For this review, take the finished solid that the model builds, in its own axes (mm). Face numbers are marked on the shaded views. Round coordinates to 2 decimals unless told otherwise and drop trailing zeros. Order: outer loops, then holes, each group sorted by start corner. A loop starts at its lowest first (then second) coordinate and runs counter-clockwise, first axis right, second up. Notation, with made-up numbers: (82.25, -9) -> (135.25, -9) arc R15 ccw to (135.25, -3) -> close; hole circle Ø9 at (83.5, 88.25). An arc over 180 degrees is marked (long way). Use a Markdown table: item, result. Add a question column.
1) Wall thickness on line 1 along X through (y, z) = (8, 0); line 2 along X through (y, z) = (8.75, 43); line 3 along X through (y, z) = (9, 0): over which ranges is each line inside the solid? List them lowest first. Write a range as [from, to].
2) Draft analysis for pull direction Z (two halves, no side actions). For the marked faces 1 and 2, state which applies: pulls with the +Z half, pulls with the -Z half, needs draft (parallel to the pull), parting line crosses it, or undercut.
3) Consider section A-A (x = 0). State the section outline as (y, z) points, plus the area to 3 significant figures.
4) Clearance check with flat-ended pins moving along their axes: P1, Ø5.5, axis at x = 72.5, y = 12.5, coming from the -Z side; P2, Ø5, axis at x = 16.5, y = 13.5, coming from the +Z side; P3, Ø5, axis at x = -97, z = 46.5, coming from the +Y side. State where each tip first meets the part, or that it passes through.
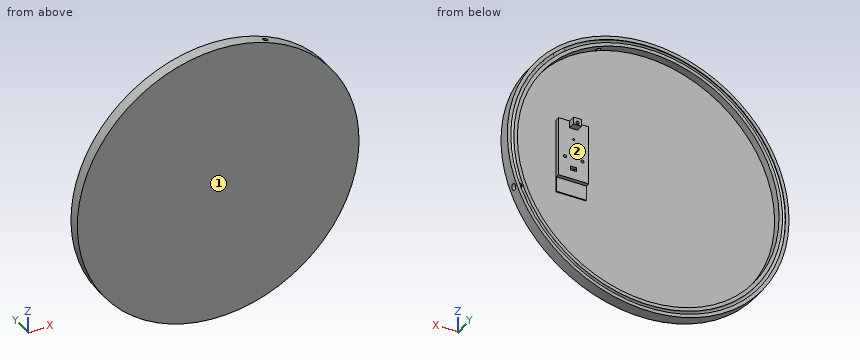
```python
from build123d import *

# Parameters (mm, degrees)
SKETCH1_R                 = 141
BOSS_EXTRUDE1_DEPTH       = 3.5
SKETCH2_R                 = 141
SKETCH2_R_2               = 131
BOSS_EXTRUDE2_DEPTH       = 8
SKETCH5_R                 = 2
CUT_EXTRUDE3_DEPTH        = 5
CUT_EXTRUDE3_DEPTH_BACK   = 15
SKETCH7_W                 = 30
SKETCH7_H                 = 75
SKETCH7_R                 = 1
BOSS_EXTRUDE3_DEPTH       = 5
SKETCH8_W                 = 8
SKETCH8_H                 = 7
BOSS_EXTRUDE4_DEPTH       = 7
SKETCH9_W                 = 6
SKETCH9_H                 = 4
CUT_EXTRUDE6_DEPTH        = 3.5
F_3_0MM_DOWEL_HOLE2_D     = 3
F_3_0MM_DOWEL_HOLE2_DEPTH = 10
F_3_0MM_DOWEL_HOLE2_TIP   = 0.901290929
F_3_0MM_DOWEL_HOLE3_D     = 3
F_3_0MM_DOWEL_HOLE3_DEPTH = 5
F_3_0MM_DOWEL_HOLE3_TIP   = 0.901290929
SKETCH10_W                = 30
SKETCH10_H                = 15
CUT_EXTRUDE7_DEPTH        = 4
SKETCH15_R                = 3
CUT_EXTRUDE9_DEPTH        = 15


with BuildPart() as part:
    # Sketch1 → Boss-Extrude1 (new body)
    with BuildSketch(Plane(origin=(0, 0, 0), x_dir=(1, 0, 0), z_dir=(0, 1, 0))):
        with Locations(Location((0, 0, 0), (0, 0, 270))):
            Circle(SKETCH1_R)
    extrude(amount=BOSS_EXTRUDE1_DEPTH)

    # Sketch2 → Boss-Extrude2 (add)
    with BuildSketch(Plane(origin=(0, 3.5, 0), x_dir=(1, 0, 0), z_dir=(0, 1, 0))):
        with Locations(Location((0, 0, 0), (0, 0, 270))):
            Circle(SKETCH2_R)
        with Locations(Location((0, 0, 0), (0, 0, 270))):
            Circle(SKETCH2_R_2, mode=Mode.SUBTRACT)
    extrude(amount=BOSS_EXTRUDE2_DEPTH)

    # Cut-Sweep1: sweep along a path in Sketch3
    with BuildLine(Plane(origin=(0, 11.5, 0), x_dir=(1, 0, 0), z_dir=(0, 1, 0))) as cut_sweep1_path:
        CenterArc((0, 0), 136, 0, 360)
    # Sketch5 → Cut-Sweep1 (sweep, cut)
    with BuildSketch(Plane(origin=(0, 0, 0), x_dir=(0.35486692076616666, 0, 0.934916824399871), z_dir=(-0.9349168243998711, 0, 0.35486692076616666))):
        with Locations((136, 10.2)):
            Circle(SKETCH5_R)
    sweep(path=cut_sweep1_path.line, mode=Mode.SUBTRACT)

    # Sketch6 → Cut-Extrude3 (cut, two sides: drawn at the far end of the back side and taken through both)
    with BuildSketch(Plane(origin=(46.48756662, 0, 122.474103996), x_dir=(-0.9349168243998711, 0, 0.3548669207661666), z_dir=(-0.3548669207661666, 0, -0.9349168243998711)).offset(-CUT_EXTRUDE3_DEPTH_BACK)):
        with BuildLine():
            Line((1, 3.599112528), (-1, 3.599112528))
            ThreePointArc((-1, 3.599112528), (-2.8, 5.399112528), (-1, 7.199112528))
            Line((-1, 7.199112528), (1, 7.199112528))
            ThreePointArc((1, 7.199112528), (2.8, 5.399112528), (1, 3.599112528))
        make_face()
    extrude(amount=CUT_EXTRUDE3_DEPTH + CUT_EXTRUDE3_DEPTH_BACK, mode=Mode.SUBTRACT)

    # Sketch7 → Boss-Extrude3 (add)
    with BuildSketch(Plane(origin=(0, 3.5, 0), x_dir=(1, 0, 0), z_dir=(0, 1, 0))):
        with Locations((72.91731325, 1.748207258)):
            Rectangle(SKETCH7_W, SKETCH7_H)
        with Locations(Location((72.91731325, -17.551792742, 0), (0, 0, 270))):
            Circle(SKETCH7_R, mode=Mode.SUBTRACT)
    extrude(amount=BOSS_EXTRUDE3_DEPTH)

    # Sketch8 → Boss-Extrude4 (add)
    with BuildSketch(Plane(origin=(0, 8.5, 0), x_dir=(1, 0, 0), z_dir=(0, 1, 0))):
        with Locations((72.91731325, -32.251792742)):
            Rectangle(SKETCH8_W, SKETCH8_H)
    extrude(amount=BOSS_EXTRUDE4_DEPTH)

    # Sketch9 → Cut-Extrude6 (cut)
    with BuildSketch(Plane(origin=(0, 8.5, 0), x_dir=(1, 0, 0), z_dir=(0, 1, 0))):
        with Locations((72.91731325, 13.248207258)):
            Rectangle(SKETCH9_W, SKETCH9_H)
    extrude(amount=-CUT_EXTRUDE6_DEPTH, mode=Mode.SUBTRACT)

    # 3.0mm Dowel Hole2
    with Locations(Plane(origin=(0, 15.5, 0), x_dir=(1, 0, 0), z_dir=(0, 1, 0))):
        with Locations((72.91731325, -31.251792742)):
            Hole(F_3_0MM_DOWEL_HOLE2_D / 2, depth=F_3_0MM_DOWEL_HOLE2_DEPTH)
            with Locations((0, 0, -(F_3_0MM_DOWEL_HOLE2_DEPTH + F_3_0MM_DOWEL_HOLE2_TIP / 2))):  # 118° drill point
                Cone(0, F_3_0MM_DOWEL_HOLE2_D / 2, F_3_0MM_DOWEL_HOLE2_TIP, mode=Mode.SUBTRACT)

    # 3.0mm Dowel Hole3
    with Locations(Plane(origin=(64.16731325, 8.5, -2.748207258), x_dir=(0, 0, 1), z_dir=(0, 1, 0))):
        with Locations((0, 0), (0, 17.5)):
            Hole(F_3_0MM_DOWEL_HOLE3_D / 2, depth=F_3_0MM_DOWEL_HOLE3_DEPTH)
            with Locations((0, 0, -(F_3_0MM_DOWEL_HOLE3_DEPTH + F_3_0MM_DOWEL_HOLE3_TIP / 2))):  # 118° drill point
                Cone(0, F_3_0MM_DOWEL_HOLE3_D / 2, F_3_0MM_DOWEL_HOLE3_TIP, mode=Mode.SUBTRACT)

    # Sketch10 → Cut-Extrude7 (cut)
    with BuildSketch(Plane(origin=(0, 8.5, 0), x_dir=(1, 0, 0), z_dir=(0, 1, 0))):
        with Locations((72.91731325, 31.748207258)):
            Rectangle(SKETCH10_W, SKETCH10_H)
    extrude(amount=-CUT_EXTRUDE7_DEPTH, mode=Mode.SUBTRACT)

    # Sketch15 → Cut-Extrude9 (cut)
    with BuildSketch(Plane(origin=(131.82327224, 0, -50.036235828), x_dir=(-0.3548669207661667, 0, -0.934916824399871), z_dir=(0.934916824399871, 0, -0.3548669207661667))):
        with Locations((0, 6.5)):
            Circle(SKETCH15_R)
    extrude(amount=-CUT_EXTRUDE9_DEPTH, mode=Mode.SUBTRACT)


solid = part.part
```
Results list:
| question | item | result |
|---|---|---|
| 1 | line 1 | [-141, -131], [57.92, 87.92], [131, 141] |
| 1 | line 2 | [-134.28, -130.47], [-127.57, -123.74], [123.74, 127.57], [130.47, 134.28] |
| 1 | line 3 | [-141, -137.6], [-134.4, -131], [131, 134.4], [137.6, 141] |
| 2 | face 1 | needs draft |
| 2 | face 2 | undercut |
| 3 | outline | (0, -141) -> (11.5, -141) -> (11.5, -137.52) arc R2 cw (long way) to (11.5, -134.48) -> (11.5, -131) -> (3.5, -131) -> (3.5, 131) -> (11.5, 131) -> (11.5, 134.48) arc R2 cw (long way) to (11.5, 137.52) -> (11.5, 141) -> (0, 141) -> close |
| 3 | area | 1,120 mm2 |
| 4 | P1 | z = -122.43 |
| 4 | P2 | z = 140.2 |
| 4 | P3 | y = 3.5 |
